The listing builds one solid part. Answer for the finished solid, in the listing's coordinates (mm). A direction names the side the tool comes from. Give positions to 0.01 mm unless a question says otherwise; leave off trailing zeros. Order: outer loops, then holes, each group sorted by start corner. A loop starts at its lowest first (then second) coordinate and runs counter-clockwise, first axis right, second up. Notation, with made-up numbers: (69.25, 61) - (116.25, 61) arc R14 ccw to (116.25, 85) - close; hole circle Ø9 at (-34, -21). An arc over 180 degrees is marked (long way). Use a Markdown table: item, result. Add a question column.
1) Find section A-A, the plane z = 20.5. Determine the outline of the cut face in (x, y).
2) Find section C-C, the plane y = -81.25. Determine the outline of the cut face in (x, z) (3 decimals).
3) For faces 1 (the face through (36, -81, 0)), 2 (the face through (59.485, -65.574, 44.219)), 3 (the face through (-4.49, -88.12, 3.22)), determine the directions among +Z, -Z, +X, -X, +Y, -Y from which every point of the face is accessible in a straight line to the end or side of a thin tool.
4) The mould has two halves that part along X. Classify faces 4 (the face through (59.46, -65.34, 14.81)), 5 (the face through (-62.04, -63.09, 50.56)), 6 (the face through (62.025, -62.903, 50.566)): released by +X, released by -X, zero draft, split by the parting line, or undercut.
5) Straight lines are drawn through the part: line 1 (X direction, y = -63.25, z = 41.5); line 2 (X direction, y = -73.5, z = 47); line 3 (Y direction, x = -18, z = 10.5). For each, find the intervals that lie inside material, in ascending order.
6) Find section D-D, the plane y = -75.5. Determine the outline of the cut face in (x, z) (3 decimals), plus the area to 3 significant figures.
7) Flat-ended cylindrical pins translate along their axes: pin 1 (10 mm diameter, centred on x = -37.5, z = 36, fed in from +Y); pin 2 (0.5 mm diameter, centred on x = 0, y = -88.5, fed in from -Z); pin 3 (1.5 mm diameter, centred on x = 33, z = 6, fed in from +Y); pin 4 (0.5 mm diameter, centred on y = -64, z = 33.5, fed in from -X). Find the tip coordinate at first contact, or state that the pin passes through.
8) Find section B-B, the plane x = -32.5. Determine the outline of the cut face in (y, z) (3 decimals), plus the area to 3 significant figures.
from build123d import *

# Parameters (mm, degrees)
F1_DEPTH = 63.5
F3_DEPTH = 127


with BuildPart() as f1:
    # F0 (on Top) → F1 (new body)
    with BuildSketch(Plane.XY):
        with BuildLine():
            Line((-61.709456, -62.217039), (-63.5, -62.217039))
            ThreePointArc((-63.5, -62.217039), (0, -88.9), (63.5, -62.217039))
            Line((63.5, -62.217039), (61.709456, -62.217039))
            ThreePointArc((61.709456, -62.217039), (0, -87.63), (-61.709456, -62.217039))
        make_face()
    extrude(amount=F1_DEPTH)

    # F2 (on Front) → F3 (cut)
    with BuildSketch(Plane.XZ):
        with BuildLine():
            ThreePointArc((-63.5, 48.26), (-62.756051, 50.056051), (-60.96, 50.8))
            Line((-60.96, 50.8), (60.96, 50.8))
            ThreePointArc((60.96, 50.8), (62.756051, 50.056051), (63.5, 48.26))
            Line((63.5, 48.26), (63.5, 63.5))
            Line((63.5, 63.5), (-63.5, 63.5))
            Line((-63.5, 63.5), (-63.5, 48.26))
        make_face()
        with BuildLine():
            Line((55.88, 45.72), (-55.88, 45.72))
            ThreePointArc((-55.88, 45.72), (-59.472102, 44.232102), (-60.96, 40.64))
            Line((-60.96, 40.64), (-60.96, 18.415))
            ThreePointArc((-60.96, 18.415), (-59.472102, 14.822898), (-55.88, 13.335))
            Line((-55.88, 13.335), (55.88, 13.335))
            ThreePointArc((55.88, 13.335), (59.472102, 14.822898), (60.96, 18.415))
            Line((60.96, 18.415), (60.96, 40.64))
            ThreePointArc((60.96, 40.64), (59.472102, 44.232102), (55.88, 45.72))
        make_face()
        with BuildLine():
            Line((63.5, 0), (63.5, 2.54))
            ThreePointArc((63.5, 2.54), (62.756051, 0.743949), (60.96, 0))
            Line((60.96, 0), (63.5, 0))
        make_face()
        with BuildLine():
            Line((-2.683826, 6.35), (-6.35, 0))
            Line((-6.35, 0), (6.35, 0))
            Line((6.35, 0), (2.683826, 6.35))
            ThreePointArc((2.683826, 6.35), (1.754121, 7.279705), (0.484121, 7.62))
            Line((0.484121, 7.62), (-0.484121, 7.62))
            ThreePointArc((-0.484121, 7.62), (-1.754121, 7.279705), (-2.683826, 6.35))
        make_face()
        with BuildLine():
            ThreePointArc((-60.96, 0), (-62.756051, 0.743949), (-63.5, 2.54))
            Line((-63.5, 2.54), (-63.5, 0))
            Line((-63.5, 0), (-60.96, 0))
        make_face()
    extrude(amount=F3_DEPTH, mode=Mode.SUBTRACT)


solid = f1.part
The answers:
| question | item | result |
|---|---|---|
| 1 | outline | (-63.5, -62.22) arc R88.9 ccw to (-60.96, -64.71) - (-60.96, -62.95) arc R87.63 cw to (-61.71, -62.22) - close; (60.96, -64.71) arc R88.9 ccw to (63.5, -62.22) - (61.71, -62.22) arc R87.63 cw to (60.96, -62.95) - close |
| 2 | outline | (-36.078, 0) - (-32.825, 0) - (-32.825, 13.335) - (-36.078, 13.335) - close; (-36.078, 45.72) - (-32.825, 45.72) - (-32.825, 50.8) - (-36.078, 50.8) - close; (32.825, 0) - (36.078, 0) - (36.078, 13.335) - (32.825, 13.335) - close; (32.825, 45.72) - (36.078, 45.72) - (36.078, 50.8) - (32.825, 50.8) - close |
| 3 | face 1 | -Z, +X, -X, +Y, -Y |
| 3 | face 2 | +Y, -Y |
| 3 | face 3 | -Z, +Y, -Y |
| 4 | face 4 | undercut |
| 4 | face 5 | released by -X |
| 4 | face 6 | released by +X |
| 5 | line 1 | -62.47 to -60.89, 60.89 to 62.47 |
| 5 | line 2 | -50.01 to -47.72, 47.72 to 50.01 |
| 5 | line 3 | -87.06 to -85.76 |
| 6 | outline | (-46.936, 0) - (-44.483, 0) - (-44.483, 13.335) - (-46.936, 13.335) - close; (-46.936, 45.72) - (-44.483, 45.72) - (-44.483, 50.8) - (-46.936, 50.8) - close; (44.483, 0) - (46.936, 0) - (46.936, 13.335) - (44.483, 13.335) - close; (44.483, 45.72) - (46.936, 45.72) - (46.936, 50.8) - (44.483, 50.8) - close |
| 6 | area | 90.3 mm2 |
| 7 | pin 1 | through |
| 7 | pin 2 | z = 7.62 |
| 7 | pin 3 | y = -80.87 |
| 7 | pin 4 | x = -61.96 |
| 8 | outline | (-82.746, 0) - (-81.38, 0) - (-81.38, 13.335) - (-82.746, 13.335) - close; (-82.746, 45.72) - (-81.38, 45.72) - (-81.38, 50.8) - (-82.746, 50.8) - close |
| 8 | area | 25.2 mm2 |
